The drawing under review shows one solid part. Ordinate dimensions are in mm from its lowest x, y, z. A direction names the side the tool comes from. Coordinates: 2 decimals unless noted, no trailing zeros. Write each loop counter-clockwise with the first axis right and the second up, starting at its lowest first coordinate (ties: lowest second). Pieces come first, ordered by that corner, then holes. Notation, with made-up numbers: (-30.75, 19.5) - (7.25, 19.5) arc R14 ccw to (7.25, 30.5) - close; hole circle Ø3 at (-31.75, 76.25). An arc over 180 degrees is marked (long way). Put each result on its own line as item: value. Start each with the question number.
Item 1: To check wall thickness, follow L1, parallel to Y at x = 26, z = 6.75 (1 decimal); L2, parallel to Z at x = 33, y = 25; L3, parallel to Y at x = 27.5, z = 7. State the ranges of each line that lie inside material, in increasing order. Write a range as [from, to].
Item 2: For pin 1 (4 mm diameter, centred on x = 64.5, z = 7, fed in from +Y), flat-tipped, find the tip position at first contact; note if it passes through.
Item 3: Consider section C-C on z = 4. Give the boundary of the cut face in (x, y).
Item 4: Consider section A-A on y = 25. Give the boundary of the cut face in (x, z).
Item 5: Machinability: for the marked faces 4 and 5, which of the approach directions +Z, -Z, +X, -X, +Y, -Y give a long, thin tool a straight path to every point of the face, cutting with its end or side? Answer none if there is none.
Item 6: Consider section B-B on x = 27.5. Give the boundary of the cut face in (y, z).
Item 7: Mouldability with a two-part tool opening along Y and no side actions: class the marked faces 1, 2 and 3 as pulls with the +Y half, pulls with the -Y half, needs draft (parallel to the pull), parting line crosses it, or undercut.
Item 8: Consider section D-D on y = 10. Give the boundary of the cut face in (x, z) (1 decimal).
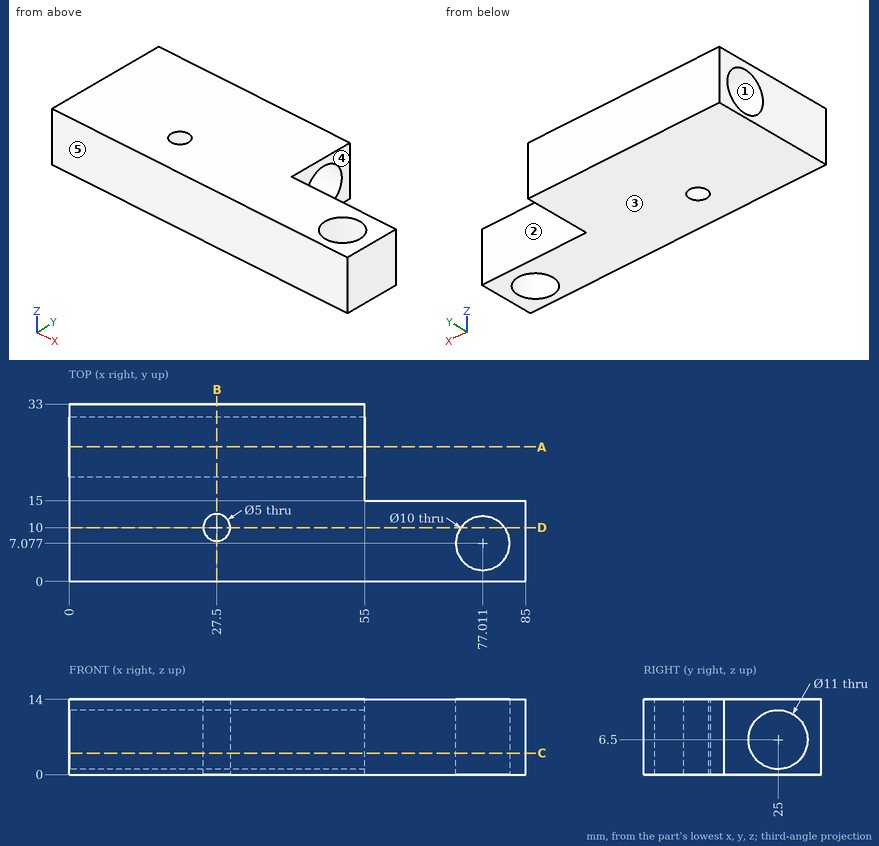
Report:
1. L1: [0, 8], [12, 19.5], [30.5, 33]
1. L2: [0, 1], [12, 14]
1. L3: [0, 7.5], [12.5, 19.52], [30.48, 33]
2. pin 1: y = 15
3. outline: (0, 0) - (85, 0) - (85, 15) - (55, 15) - (55, 20.1) - (0, 20.1) - close; (0, 29.9) - (55, 29.9) - (55, 33) - (0, 33) - close; hole circle Ø5 at (27.5, 10); hole circle Ø10 at (77.01, 7.08)
4. outline: (0, 0) - (55, 0) - (55, 1) - (0, 1) - close; (0, 12) - (55, 12) - (55, 14) - (0, 14) - close
5. face 4: +Z, -Z, +X, +Y
5. face 5: +Z, -Z, +X, -X, -Y
6. outline: (0, 0) - (7.5, 0) - (7.5, 14) - (0, 14) - close; (12.5, 0) - (33, 0) - (33, 14) - (12.5, 14) - close; hole circle Ø11 at (25, 6.5)
7. face 1: undercut
7. face 2: pulls with the +Y half
7. face 3: needs draft
8. outline: (0, 0) - (25, 0) - (25, 14) - (0, 14) - close; (30, 0) - (73, 0) - (73, 14) - (30, 14) - close; (81.1, 0) - (85, 0) - (85, 14) - (81.1, 14) - close
